Model file for the job. Use its own axes, mm. Face numbers are marked on the shaded views. Coordinates: 2 decimals unless noted, no trailing zeros. Loops run counter-clockwise (first coordinate to the right, second up) from the corner with the lowest first, then second, coordinate; pieces in that order, holes last. Notation, with made-up numbers: (44, 70) -> (58, 70) arc R23 ccw to (58, 100) -> close; hole circle Ø11 at (-20.5, 12.5). An arc over 180 degrees is marked (long way). Use one line per item in the form item = value.
```python
from build123d import *

# Parameters (mm, degrees)
SKETCH4_R           = 2.5
BOSS_EXTRUDE1_DEPTH = 2
FILLET1_R           = 2
FILLET2_R           = 1


with BuildPart() as part:
    # Sketch3 → Revolve1 (revolve)
    with BuildSketch(Plane.XY, mode=Mode.PRIVATE) as revolve1_sk:
        with BuildLine():
            Line((0, 0), (0, 22.313068229))
            ThreePointArc((0, 22.313068229), (-1.541624675, 27.064446646), (2.5, 30))
            Line((2.5, 30), (2.5, 0))
            Line((2.5, 0), (0, 0))
        make_face()
    revolve(revolve1_sk.sketch.rotate(Axis((2.5, 0, 0), (0, 1, 0)), 180), axis=Axis((2.5, 0, 0), (0, 1, 0)))

    # Sketch4 → Boss-Extrude1 (add)
    with BuildSketch(Plane.XZ):
        with BuildLine():
            Line((9.589249496, 0), (9.589249496, -45))
            ThreePointArc((9.589249496, -45), (2.589249496, -52), (-4.410750504, -45))
            Line((-4.410750504, -45), (-4.410750504, 0))
            ThreePointArc((-4.410750504, 0), (2.589249496, 7), (9.589249496, 0))
        make_face()
        with Locations(Location((2.589249496, -45, 0), (0, 0, 270))):
            Circle(SKETCH4_R, mode=Mode.SUBTRACT)
    extrude(amount=-BOSS_EXTRUDE1_DEPTH)

    # Fillet1
    fillet1_edges = [part.edges().sort_by_distance(p)[0] for p in [
        (0, 2, 0),
    ]]
    fillet(fillet1_edges, radius=FILLET1_R)

    # Fillet2
    fillet2_edges = [part.edges().sort_by_distance(p)[0] for p in [
        (0, 22.313068229, 0),
    ]]
    fillet(fillet2_edges, radius=FILLET2_R)


solid = part.part
```
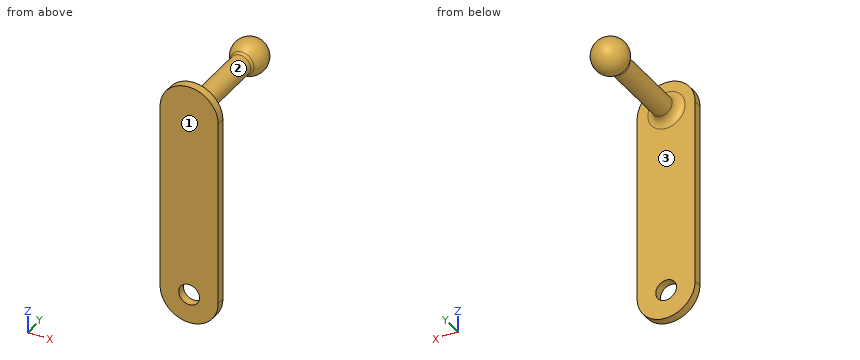
Q1. Mould opens along Y. For the marked faces 1, 2 and 3 say: released by +Y, released by -Y, zero draft, split by the parting line, or undercut.
Result:
face_1 = released by -Y
face_2 = undercut
face_3 = released by +Y
Q2. Band-saw the part on A-A, the plane y = 13.75. Write the cut outline in (x, z).
Result:
outline = circle Ø5 at (2.5, 0)
Q3. Band-saw the part on B-B, the plane z = -12. Write the cut outline in (x, y).
Result:
outline = (-4.41, 0) -> (9.59, 0) -> (9.59, 2) -> (-4.41, 2) -> close
Q4. Pin check, flat tips, straight feed: pin 1 Ø5 at (x, y) = (1, 12.5) entering from +Z; pin 2 Ø3 at (x, y) = (6, 20) entering from -Z; pin 3 Ø4 at (x, y) = (5.5, 25.5) entering from -Z. Stop position of each tip, or through.
Result:
pin_1 = 2.5
pin_2 = -1.5
pin_3 = -4.13
Q5. Band-saw the part on C-C, the plane y = 25. Write the cut outline in (x, z), and give its area (3 significant figures).
Result:
outline = circle Ø8.37 at (2.5, 0)
area = 55.0 mm2
Q6. Wall check: line 1 along X through (y, z) = (0.95, -45); line 2 along Y through (x, z) = (-2.25, -43.5); line 3 along Y through (x, z) = (5, 3). Give the ranges that are in metal, low to high.
Result:
line_1 = -4.41 to 0.09, 5.09 to 9.59
line_2 = 0 to 2
line_3 = 0 to 2.09, 24.07 to 27.43
